```python
from build123d import *

# Parameters (mm, degrees)
SKETCH1_R               = 10
BOSS_EXTRUDE1_DEPTH     = 1
SKETCH2_R               = 10
BOSS_EXTRUDE2_DEPTH     = 3
BOSS_EXTRUDE2_TAPER     = 4
SKETCH3_R               = 9.790219564
BOSS_EXTRUDE3_DEPTH     = 2
BOSS_EXTRUDE3_TAPER     = 3
SKETCH4_R               = 9.685404006
BOSS_EXTRUDE4_DEPTH     = 3
BOSS_EXTRUDE4_TAPER     = 1
SKETCH5_R               = 9.633038811
BOSS_EXTRUDE5_DEPTH     = 14
CUT_EXTRUDE1_DEPTH      = 13
CUT_EXTRUDE1_DEPTH_BACK = 13
SKETCH6_W               = 17.15
SKETCH6_H               = 11
CUT_EXTRUDE2_DEPTH      = 13
CUT_EXTRUDE2_DEPTH_BACK = 13
SKETCH8_W               = 12
SKETCH8_H               = 11
CUT_EXTRUDE3_DEPTH      = 13
SKETCH9_R               = 1.25
CUT_EXTRUDE4_DEPTH      = 11
CHAMFER1_SIZE           = 4
CHAMFER1_SIZE_2         = 3


with BuildPart() as part:
    # Sketch1 → Boss-Extrude1 (new body)
    with BuildSketch(Plane.XY):
        Circle(SKETCH1_R)
    extrude(amount=BOSS_EXTRUDE1_DEPTH)

    # Sketch2 → Boss-Extrude2 (add)
    with BuildSketch(Plane.XY.offset(1)):
        Circle(SKETCH2_R)
    extrude(amount=BOSS_EXTRUDE2_DEPTH, taper=BOSS_EXTRUDE2_TAPER)

    # Sketch3 → Boss-Extrude3 (add)
    with BuildSketch(Plane.XY.offset(4)):
        Circle(SKETCH3_R)
    extrude(amount=BOSS_EXTRUDE3_DEPTH, taper=BOSS_EXTRUDE3_TAPER)

    # Sketch4 → Boss-Extrude4 (add)
    with BuildSketch(Plane.XY.offset(6)):
        Circle(SKETCH4_R)
    extrude(amount=BOSS_EXTRUDE4_DEPTH, taper=BOSS_EXTRUDE4_TAPER)

    # Sketch5 → Boss-Extrude5 (add)
    with BuildSketch(Plane.XY.offset(9)):
        Circle(SKETCH5_R)
    extrude(amount=BOSS_EXTRUDE5_DEPTH)

    # Sketch6 → Cut-Extrude1 (cut, two sides: drawn at the far end of the back side and taken through both)
    with BuildSketch(Plane(origin=(0, 0, 0), x_dir=(0, 0, -1), z_dir=(1, 0, 0)).offset(-CUT_EXTRUDE1_DEPTH_BACK)):
        with Locations((-17.575, 0)):
            Rectangle(SKETCH6_W, SKETCH6_H)
    extrude(amount=CUT_EXTRUDE1_DEPTH + CUT_EXTRUDE1_DEPTH_BACK, mode=Mode.SUBTRACT)

    # Sketch7 → Cut-Extrude2 (cut, two sides: drawn at the far end of the back side and taken through both)
    with BuildSketch(Plane(origin=(0, 0, 0), x_dir=(1, 0, 0), z_dir=(0, 1, 0)).offset(-CUT_EXTRUDE2_DEPTH_BACK)):
        with BuildLine():
            Line((-7.9085673, -9), (-9.6485673, -9))
            Line((-9.6485673, -9), (-9.6485673, -28.451581468))
            Line((-9.6485673, -28.451581468), (9.633038811, -28.451581468))
            Line((9.633038811, -28.451581468), (9.633038811, -9))
            Line((9.633038811, -9), (5.5714327, -9))
            Line((5.5714327, -9), (5.243186995, -16.36))
            ThreePointArc((5.243186995, -16.36), (2.198477753, -21.139438677), (-3.154241182, -23))
            Line((-3.154241182, -23), (-7.324241182, -23))
            Line((-7.324241182, -23), (-7.9085673, -9))
        make_face()
    extrude(amount=CUT_EXTRUDE2_DEPTH + CUT_EXTRUDE2_DEPTH_BACK, mode=Mode.SUBTRACT)

    # Sketch8 → Cut-Extrude3 (cut)
    with BuildSketch(Plane(origin=(0, 0, 0), x_dir=(-1, 0, 0), z_dir=(0, 0, -1))):
        Rectangle(SKETCH8_W, SKETCH8_H)
    extrude(amount=-CUT_EXTRUDE3_DEPTH, mode=Mode.SUBTRACT)

    # Sketch9 → Cut-Extrude4 (cut, symmetric)
    with BuildSketch(Plane(origin=(0, 0, 0), x_dir=(1, 0, 0), z_dir=(0, 1, 0))):
        with Locations(Location((-2.9085673, -18, 0), (0, 0, 270))):
            Circle(SKETCH9_R)
    extrude(amount=CUT_EXTRUDE4_DEPTH, both=True, mode=Mode.SUBTRACT)

    # Chamfer1
    # the kernel refuses this chamfer: 4, 3 mm, written as the material it takes off along each edge
    with BuildSketch(Plane(origin=(0, 0, 9), x_dir=(-0.4396306058143097, 0.8981786740016393, 0), z_dir=(-0.8981786740016393, -0.4396306058143097, 0))) as chamfer1_piece_1_section:
        Polygon((9.633038811 - CHAMFER1_SIZE, 0), (9.633038811 + CHAMFER1_SIZE_2 * 0.0174524064373, CHAMFER1_SIZE_2 * 0.999847695156), (9.633038811, 0), align=None)
    chamfer1_piece_1 = revolve(axis=Axis((0, 0, 9), (0, 0, -1)), revolution_arc=116.080314714, mode=Mode.PRIVATE)
    chamfer1_piece_1 = split(chamfer1_piece_1, bisect_by=Plane(origin=(5.560372923, 0, 9.247984855), z_dir=(0.9990069635270564, 0, 0.04455431319693658)), keep=Keep.TOP, mode=Mode.PRIVATE)
    add(chamfer1_piece_1, mode=Mode.SUBTRACT)
    with BuildSketch(Plane(origin=(0, 0, 9), x_dir=(1, 0, 0), z_dir=(0, 1, 0))) as chamfer1_piece_2_section:
        Polygon((9.633038811 - CHAMFER1_SIZE, 0), (9.633038811 + CHAMFER1_SIZE_2 * 0.0174524064373, CHAMFER1_SIZE_2 * 0.999847695156), (9.633038811, 0), align=None)
    chamfer1_piece_2 = revolve(axis=Axis((0, 0, 9), (0, 0, -1)), revolution_arc=116.080314714, mode=Mode.PRIVATE)
    chamfer1_piece_2 = split(chamfer1_piece_2, bisect_by=Plane(origin=(5.560372923, 0, 9.247984855), z_dir=(0.9990069635270564, 0, 0.04455431319693658)), keep=Keep.TOP, mode=Mode.PRIVATE)
    add(chamfer1_piece_2, mode=Mode.SUBTRACT)


solid = part.part
```
Geometry check sheet. Reference: the model listing, model coordinates, mm. A direction names the side the tool comes from. Give positions to 0.01 mm unless a question says otherwise; leave off trailing zeros. Loops run counter-clockwise (first coordinate to the right, second up) from the corner with the lowest first, then second, coordinate; pieces in that order, holes last. Notation, with made-up numbers: M 68.5,54.25 L 108.5,54.25 A5 ccw 108.5,59.25 Z; hole C -18.5,31.25 d7. An arc over 180 degrees is marked long. Answer as CSV lines item,"result".
Item 1: Material ranges on line 1 (Y direction, x = 5.25, z = 6.25); line 2 (X direction, y = 8, z = 18); line 3 (Y direction, x = 1.25, z = 4.5), recorded low to high.
Values:
line 1,"y = -8.13 to -5.5, 5.5 to 8.13"
line 2,"x = -5.37 to -4.16, -1.66 to 4.68"
line 3,"y = -9.68 to -5.5, 5.5 to 9.68"
Item 2: Depth check by flat-ended pin: P1, Ø3, axis at x = -2.91, z = 18, coming from the -Y side; P2, Ø7, axis at x = -2, z = 10.5, coming from the +Y side; P3, Ø10, axis at y = -1, z = 8, coming from the +X side. Enter the tip coordinate at first touch or a pass-through.
Values:
P1,"stops at y = -9.53"
P2,"stops at y = 9.66"
P3,"stops at x = 9.85"
Item 3: Access from +Z, -Z, +X, -X, +Y, -Y to the whole of each face (thin tool, end or side, straight path). Record for faces 4 (the conical face through (-9.65, 0.42, 7.52)), 5 (the flat face through (-7, 0, 9)), 6 (the flat face through (-6, 0, 4)).
Values:
face 4,"+Z"
face 5,"+Z, +X, -X"
face 6,"+Z, -Z"
Item 4: Release check for a two-part mould opening along Z. For faces 1 (the conical face through (-1.282, 9.763, 3.188)), 2 (the flat face through (-1, -5.5, 11)), 3 (the cylindrical face through (-1.67, -7.47, 17.84)) record: pulls with the +Z half, pulls with the -Z half, needs draft (parallel to the pull), parting line crosses it, or undercut.
Values:
face 1,"pulls with the +Z half"
face 2,"needs draft"
face 3,"undercut"
Item 5: Cross-section at A-A on z = 14.75. Record the cut outline in (x, y) (3 decimals).
Values:
outline,"M -7.669,-5.83 A9.633 ccw 5.315,-8.034 L 5.315,-5.5 L -7.669,-5.5 Z; M -7.669,5.5 L 5.315,5.5 L 5.315,8.034 A9.633 ccw -7.669,5.83 Z"
Item 6: Cross-section at B-B on z = 18. Record the cut outline in (x, y).
Values:
outline,"M -7.53,-6 A9.63 ccw -4.16,-8.69 L -4.16,-5.5 L -7.53,-5.5 Z; M -7.53,5.5 L -4.16,5.5 L -4.16,8.69 A9.63 ccw -7.53,6 Z; M -1.66,-9.49 A9.63 ccw 4.68,-8.42 L 4.68,-5.5 L -1.66,-5.5 Z; M -1.66,5.5 L 4.68,5.5 L 4.68,8.42 A9.63 ccw -1.66,9.49 Z"
